Part model, mm, in its own coordinate system. A direction names the side the tool comes from. Coordinates: 2 decimals unless noted, no trailing zeros. Order: outer loops, then holes, each group sorted by start corner. A loop starts at its lowest first (then second) coordinate and runs counter-clockwise, first axis right, second up. Notation, with made-up numbers: M 64.5,78 L 111.5,78 A28 ccw 111.5,116 Z; hole C 62.25,84.5 d3. An arc over 180 degrees is marked long. Answer in a Markdown table with one row per item. Add a question column.
from build123d import *

# Parameters (mm, degrees)
SKETCH1_R           = 2.2
BOSS_EXTRUDE1_DEPTH = 5
SKETCH2_R           = 1
CUT_EXTRUDE1_DEPTH  = 153.151240547


with BuildPart() as part:
    # Sketch1 → Boss-Extrude1 (new body)
    with BuildSketch(Plane.XY):
        with BuildLine():
            Line((0, 105), (0, 110))
            Line((0, 110), (100, 110))
            Line((100, 110), (100, 105))
            ThreePointArc((100, 105), (103.535533906, 103.535533906), (105, 100))
            Line((105, 100), (105, 20))
            Line((105, 20), (100, 20))
            Line((100, 20), (0, 20))
            Line((0, 20), (-5, 20))
            Line((-5, 20), (-5, 100))
            ThreePointArc((-5, 100), (-3.535533906, 103.535533906), (0, 105))
        make_face()
        with Locations((0, 100)):
            Circle(SKETCH1_R, mode=Mode.SUBTRACT)
        with Locations((0, 30)):
            Circle(SKETCH1_R, mode=Mode.SUBTRACT)
        with Locations(Location((100, 30, 0), (0, 0, 180))):
            Circle(SKETCH1_R, mode=Mode.SUBTRACT)
        with Locations(Location((100, 100, 0), (0, 0, 180))):
            Circle(SKETCH1_R, mode=Mode.SUBTRACT)
        Polygon((0, 85), (2.5, 85), (2.5, 75), (0, 75), (-2.5, 75), (-2.5, 85), align=None, mode=Mode.SUBTRACT)
        Polygon((102.5, 75), (100, 75), (97.5, 75), (97.5, 85), (100, 85), (102.5, 85), align=None, mode=Mode.SUBTRACT)
    extrude(amount=BOSS_EXTRUDE1_DEPTH)

    # Sketch2 → Cut-Extrude1 (cut, through all)
    with BuildSketch(Plane.XY.offset(5)):
        with Locations((18, 94)):
            Circle(SKETCH2_R)
        with Locations((37, 94)):
            Circle(SKETCH2_R)
        with Locations((18, 77.5)):
            Circle(SKETCH2_R)
        with Locations((37, 77.5)):
            Circle(SKETCH2_R)
        with Locations(Location((63, 77.5, 0), (0, 0, 180))):
            Circle(SKETCH2_R)
        with Locations(Location((82, 77.5, 0), (0, 0, 180))):
            Circle(SKETCH2_R)
        with Locations(Location((63, 94, 0), (0, 0, 180))):
            Circle(SKETCH2_R)
        with Locations(Location((82, 94, 0), (0, 0, 180))):
            Circle(SKETCH2_R)
    extrude(amount=-CUT_EXTRUDE1_DEPTH, mode=Mode.SUBTRACT)


solid = part.part
(1) Slice it at A-A (y = 82). List the corners of the cut face in (x, z).
(2) Slice it at B-B (y = 30). List the corners of the cut face in (x, z).
(3) 3-axis set-ups, long thin cutter, end or side, ignore diameter. For faces 5 (the cylindrical face through (-4, 103, 2)), 6 (the flat face through (0, 75, 2)): which of +Z, -Z, +X, -X, +Y, -Y reach the whole face in a straight line?
(4) Pull direction Y, two halves, no side cores. Call faces 1 (the flat face through (-2.5, 80, 2)), 2 (the flat face through (51, 66, 0)), 3 (the flat face through (49, 110, 2)), 4 (the cylindrical face through (-0.477, 27.852, 2.465)): pulls with the +Y half, pulls with the -Y half, needs draft (parallel to the pull), parting line crosses it, or undercut.
(5) Wall check: line 1 (X direction, y = 76, z = 1.65); line 2 (Y direction, x = 37, z = 1.55); line 3 (X direction, y = 94, z = 4). Give the ranges that are in metal, low to high.
Computed:
| question | item | result |
|---|---|---|
| 1 | outline | M -5,0 L -2.5,0 L -2.5,5 L -5,5 Z; M 2.5,0 L 97.5,0 L 97.5,5 L 2.5,5 Z; M 102.5,0 L 105,0 L 105,5 L 102.5,5 Z |
| 2 | outline | M -5,0 L -2.2,0 L -2.2,5 L -5,5 Z; M 2.2,0 L 97.8,0 L 97.8,5 L 2.2,5 Z; M 102.2,0 L 105,0 L 105,5 L 102.2,5 Z |
| 3 | face 5 | +Z, -Z, -X, +Y |
| 3 | face 6 | +Z, -Z |
| 4 | face 1 | undercut |
| 4 | face 2 | needs draft |
| 4 | face 3 | pulls with the +Y half |
| 4 | face 4 | undercut |
| 5 | line 1 | x = -5 to -2.5, 2.5 to 97.5, 102.5 to 105 |
| 5 | line 2 | y = 20 to 76.5, 78.5 to 93, 95 to 110 |
| 5 | line 3 | x = -5 to 17, 19 to 36, 38 to 62, 64 to 81, 83 to 105 |
